The listing builds one solid part. Answer for the finished solid, in the listing's coordinates (mm). A direction names the side the tool comes from. Give positions to 0.01 mm unless a question says otherwise; leave off trailing zeros. Loops run counter-clockwise (first coordinate to the right, second up) from the corner with the lowest first, then second, coordinate; pieces in that order, holes last. Notation, with made-up numbers: M 49.25,20.25 L 96.25,20.25 A23 cw 96.25,54.25 Z; hole C 57,-31.75 d1. An arc over 180 degrees is marked long. Return JSON: item names as keys, results as strings.
from build123d import *

# Parameters (mm, degrees)
BOSS_EXTRU_1_DEPTH      = 8
ESQUISSE2_R             = 2
ENL_V_MAT_EXTRU_1_DEPTH = 15
ENL_V_START             = -10
ESQUISSE3_R             = 2
ENL_V_MAT_EXTRU_2_DEPTH = 10
ESQUISSE4_R             = 2
ENL_V_MAT_EXTRU_3_DEPTH = 10
CHANFREIN1_SIZE         = 2.5
ESQUISSE5_W             = 50
ESQUISSE5_H             = 8
ENL_V_MAT_EXTRU_4_DEPTH = 2
ESQUISSE6_W             = 19
ESQUISSE6_H             = 8
BOSS_EXTRU_2_DEPTH      = 10
CONG_1_R                = 3.5
ESQUISSE7_R             = 2
ENL_V_MAT_EXTRU_5_DEPTH = 82.808975418


with BuildPart() as part:
    # Esquisse1 → Boss.-Extru.1 (new body)
    with BuildSketch(Plane(origin=(0, 0, 0), x_dir=(1, 0, 0), z_dir=(0, 1, 0))):
        Polygon((-57.148145082, 46.041666667), (-7.148145082, 46.041666667), (-7.148145082, 16.041666667), (-7.148145082, -1.958333333), (-16.148145082, -1.958333333), (-16.148145082, 10.041666667), (-27.148145082, 10.041666667), (-27.148145082, -1.958333333), (-37.148145082, -1.958333333), (-37.148145082, 10.041666667), (-48.148145082, 10.041666667), (-57.148145082, 10.041666667), align=None)
    extrude(amount=BOSS_EXTRU_1_DEPTH)

    # Esquisse2 → Enlèv. mat.-Extru.1 (cut)
    with BuildSketch(Plane.XY.offset(1.958333333)):
        with Locations((-52.148145082, 4)):
            Circle(ESQUISSE2_R)
        with Locations((-12.148145082, 4)):
            Circle(ESQUISSE2_R)
        with Locations((-32.148145082, 4)):
            Circle(ESQUISSE2_R)
    extrude(amount=-ENL_V_MAT_EXTRU_1_DEPTH, mode=Mode.SUBTRACT)

    # Esquisse3 → Enlèv. mat.-Extru.2 (cut)
    with BuildSketch(Plane(origin=(0, 0, -46.041666667), x_dir=(-1, 0, 0), z_dir=(0, 0, -1)).offset(ENL_V_START)):
        with Locations(Location((12.148145082, 4, 0), (0, 0, 180))):
            Circle(ESQUISSE3_R)
        with Locations(Location((52.148145082, 4, 0), (0, 0, 180))):
            Circle(ESQUISSE3_R)
    extrude(amount=ENL_V_MAT_EXTRU_2_DEPTH, mode=Mode.SUBTRACT)

    # Esquisse4 → Enlèv. mat.-Extru.3 (cut)
    with BuildSketch(Plane(origin=(0, 8, 0), x_dir=(1, 0, 0), z_dir=(0, 1, 0))):
        with Locations(Location((-52.148145082, 23.041666667, 0), (0, 0, 270))):
            Circle(ESQUISSE4_R)
        with Locations(Location((-12.148145082, 23.041666667, 0), (0, 0, 270))):
            Circle(ESQUISSE4_R)
    extrude(amount=-ENL_V_MAT_EXTRU_3_DEPTH, mode=Mode.SUBTRACT)

    # Chanfrein1
    chanfrein1_edges = [part.edges().sort_by_distance(p)[0] for p in [
        (-52.148145082, 0, -25.041666667),
        (-12.148145082, 0, -25.041666667),
    ]]
    chamfer(chanfrein1_edges, length=CHANFREIN1_SIZE)

    # Esquisse5 → Enlèv. mat.-Extru.4 (cut)
    with BuildSketch(Plane(origin=(0, 8, 0), x_dir=(1, 0, 0), z_dir=(0, 1, 0))):
        with Locations((-32.148145082, 23.041666667)):
            Rectangle(ESQUISSE5_W, ESQUISSE5_H)
    extrude(amount=-ENL_V_MAT_EXTRU_4_DEPTH, mode=Mode.SUBTRACT)

    # Esquisse6 → Boss.-Extru.2 (add)
    with BuildSketch(Plane.ZY.offset(57.148145082)):
        with Locations((-9.541666667, 4)):
            Rectangle(ESQUISSE6_W, ESQUISSE6_H)
    extrude(amount=BOSS_EXTRU_2_DEPTH)

    # Congé1
    cong_1_edges = [part.edges().sort_by_distance(p)[0] for p in [
        (-16.148145082, 4, -10.041666667),
        (-27.148145082, 4, -10.041666667),
        (-37.148145082, 4, -10.041666667),
        (-57.148145082, 4, -10.041666667),
        (-57.148145082, 3, -19.041666667),
    ]]
    fillet(cong_1_edges, radius=CONG_1_R)

    # Esquisse7 → Enlèv. mat.-Extru.5 (cut, through all)
    with BuildSketch(Plane(origin=(0, 8, 0), x_dir=(1, 0, 0), z_dir=(0, 1, 0))):
        with Locations(Location((-62.148145082, 5.041666667, 0), (0, 0, 270))):
            Circle(ESQUISSE7_R)
    extrude(amount=-ENL_V_MAT_EXTRU_5_DEPTH, mode=Mode.SUBTRACT)


solid = part.part
(1) Given pin 1 (6.5 mm diameter, centred on x = -33, z = -23.5, fed in from +Y); pin 2 (5 mm diameter, centred on x = -12.15, z = -23.04, fed in from -Y); pin 3 (3 mm diameter, centred on x = -21, y = 6, fed in from +Z), each flat-ended and moving along its own axis, determine where each tip first touches the part or whether it passes through.
Values follow:
{"pin 1": "y = 6", "pin 2": "y = 2", "pin 3": "z = -10.04"}
(2) The part is cut by section B-B (z = -43). Determine the outline of the cut face in (x, y), and give its area (3 significant figures).
Values follow:
{"outline": "M -57.15,0 L -7.15,0 L -7.15,8 L -57.15,8 Z; hole C -52.15,4 d4; hole C -12.15,4 d4", "area": "375 mm²"}
(3) The part is cut by section A-A (x = -43). Determine the outline of the cut face in (y, z), and give its area (3 significant figures).
Values follow:
{"outline": "M 0,-46.04 L 8,-46.04 L 8,-27.04 L 6,-27.04 L 6,-19.04 L 8,-19.04 L 8,-10.04 L 0,-10.04 Z", "area": "272 mm²"}
(4) Determine the mould class of faces 1 (the conical face through (-12.05, 2.38, -25.16)), 2 (the cylindrical face through (-58.2, 3.04, -20.04)), 3 (the cylindrical face through (-54.146, 4.088, -11.521)), 4 (the cylindrical face through (-56.1, 6.68, -9.04)) for opening direction Z: released by +Z, released by -Z, zero draft, split by the parting line, or undercut.
Values follow:
{"face 1": "undercut", "face 2": "released by -Z", "face 3": "zero draft", "face 4": "released by +Z"}
(5) The part is cut by section C-C (y = 4). Give the number of separate pieces and of enclosed holes in the cut face, and give its area (3 significant figures).
Values follow:
{"separate pieces": "1", "enclosed holes": "3", "area": "1,980 mm²"}
(6) Straight lines are drawn through the part: line 1 along Z through (x, y) = (-41.5, 6.5); line 2 along Z through (x, y) = (-34.5, 6.75); line 3 along X through (y, z) = (5.25, -13). For each, find the intervals that lie inside material, in ascending order.
Values follow:
{"line 1": "-46.04 to -27.04, -19.04 to -10.04", "line 2": "-46.04 to -27.04, -19.04 to 1.96", "line 3": "-67.15 to -53.71, -50.59 to -33.71, -30.59 to -13.71, -10.59 to -7.15"}
(7) A tool of negligible diameter and unlimited length cuts with its end or side. For faces 5 (the flat face through (-57.148, 4, -3)), 6 (the flat face through (-57.148, 4, -34)), 7 (the flat face through (-43.7, 6.4, -19.042)), from which of +Z, -Z, +X, -X, +Y, -Y can it reach the whole face along a straight path? Write none if from no direction.
Values follow:
{"face 5": "+Z, +Y, -Y", "face 6": "-Z, -X, +Y, -Y", "face 7": "-X, +Y"}
(8) The part is cut by section D-D (x = -36.5). Determine the outline of the cut face in (y, z), and give its area (3 significant figures).
Values follow:
{"outline": "M 0,-46.04 L 8,-46.04 L 8,-27.04 L 6,-27.04 L 6,-19.04 L 8,-19.04 L 8,1.96 L 0,1.96 Z", "area": "368 mm²"}
